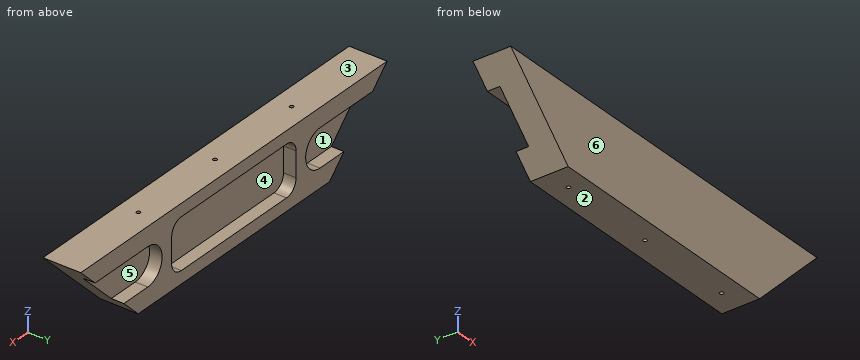
```python
from build123d import *

# Parameters (mm, degrees)
BOSS_EXTRUDE1_DEPTH = 15
CUT_EXTRUDE1_DEPTH  = 5
SKETCH3_R           = 0.75
CUT_EXTRUDE2_DEPTH  = 30
CUT_EXTRUDE3_DEPTH  = 5


with BuildPart() as part:
    # Sketch1 → Boss-Extrude1 (new body)
    with BuildSketch(Plane(origin=(0, 0, 0), x_dir=(1, 0, 0), z_dir=(0, 1, 0))):
        Polygon((0, 0), (160, 0), (130, 30), (30, 30), align=None)
    extrude(amount=BOSS_EXTRUDE1_DEPTH)

    # Sketch2 → Cut-Extrude1 (cut)
    with BuildSketch(Plane(origin=(0, 15, 0), x_dir=(1, 0, 0), z_dir=(0, 1, 0))):
        with BuildLine():
            Line((-5, 22.5), (35, 22.5))
            ThreePointArc((35, 22.5), (42.5, 15), (35, 7.5))
            Line((35, 7.5), (-5, 7.5))
            ThreePointArc((-5, 7.5), (-12.5, 15), (-5, 22.5))
        make_face()
        with BuildLine():
            Line((165, 22.5), (125, 22.5))
            ThreePointArc((125, 22.5), (117.5, 15), (125, 7.5))
            Line((125, 7.5), (165, 7.5))
            ThreePointArc((165, 7.5), (172.5, 15), (165, 22.5))
        make_face()
    extrude(amount=-CUT_EXTRUDE1_DEPTH, mode=Mode.SUBTRACT)

    # Sketch3 → Cut-Extrude2 (cut)
    with BuildSketch(Plane.XY):
        with Locations((80, 7.5)):
            Circle(SKETCH3_R)
        with Locations((40, 7.5)):
            Circle(SKETCH3_R)
        with Locations((120, 7.5)):
            Circle(SKETCH3_R)
    extrude(amount=-CUT_EXTRUDE2_DEPTH, mode=Mode.SUBTRACT)

    # Sketch4 → Cut-Extrude3 (cut)
    with BuildSketch(Plane(origin=(0, 15, 0), x_dir=(1, 0, 0), z_dir=(0, 1, 0))):
        with BuildLine():
            Line((52.5, 25), (107.5, 25))
            ThreePointArc((107.5, 25), (111.035533906, 23.535533906), (112.5, 20))
            Line((112.5, 20), (112.5, 10))
            ThreePointArc((112.5, 10), (111.035533906, 6.464466094), (107.5, 5))
            Line((107.5, 5), (52.5, 5))
            ThreePointArc((52.5, 5), (48.964466094, 6.464466094), (47.5, 10))
            Line((47.5, 10), (47.5, 20))
            ThreePointArc((47.5, 20), (48.964466094, 23.535533906), (52.5, 25))
        make_face()
    extrude(amount=-CUT_EXTRUDE3_DEPTH, mode=Mode.SUBTRACT)


solid = part.part
```
CAD build for the part. Positions are in the model's coordinates, mm. Face numbers are marked on the shaded views. A direction names the side the tool comes from. Coordinates: 2 decimals unless noted, no trailing zeros. Order: outer loops, then holes, each group sorted by start corner. A loop starts at its lowest first (then second) coordinate and runs counter-clockwise, first axis right, second up. Notation, with made-up numbers: M 8.25,-7 L 20.25,-7 A14 cw 20.25,7 Z; hole C 76.5,62.25 d6. An arc over 180 degrees is marked long. Write each question's results on one line, items separated by ' | '. Start each with the question number.
Q1. Drill centre lines: probe 1 along Y at (x, z) = (80, -12.25); probe 2 along Y at (x, z) = (40, -22); probe 3 along Z at (x, y) = (95, 10.25). Where is each one in solid material? Low to high. Write a range as from..to.
Q2. Cut at D-D (z = -15). List the corners of the cut face in (x, y).
Q3. Cut at C-C (z = -26.5). List the corners of the cut face in (x, y).
Q4. Pull direction Z, two halves, no side cores. Call the marked faces 1, 2 and 3: +Z half, -Z half, draft (parallel to the pull), parting line (faces both ways), or undercut.
Q5. Which spindle directions (+Z, -Z, +X, -X, +Y, -Y) get a long thin tool onto all of the face, cutting with end or side? Do the marked faces 4, 5 and 6. Say none if no direction does.
Q6. Cut at B-B (x = 93). List the corners of the cut face in (y, z).
Q7. Flat gauge pins, fed straight in: P1, Ø2, axis at y = 10.5, z = -10, coming from the -X side; P2, Ø5, axis at y = 11, z = -5.5, coming from the -X side; P3, Ø1.5, axis at x = 136, y = 12, coming from the -Z side; P4, Ø5.5, axis at x = 31, y = 13, coming from the +Z side. Where does each tip first touch, or does it go through?
Q8. Cut at A-A (z = -2.5). List the corners of the cut face in (x, y), then the cut area to 3 significant figures.
Found:
1) probe 1: 0..6.75, 8.25..10 | probe 2: 0..6.75, 8.25..15 | probe 3: -30..-25, -5..0
2) outline: M 15,0 L 145,0 L 145,10 L 117.5,10 L 117.5,15 L 112.5,15 L 112.5,10 L 47.5,10 L 47.5,15 L 42.5,15 L 42.5,10 L 15,10 Z; hole C 40,7.5 d1.5; hole C 80,7.5 d1.5; hole C 120,7.5 d1.5
3) outline: M 26.5,0 L 133.5,0 L 133.5,15 L 26.5,15 Z; hole C 40,7.5 d1.5; hole C 80,7.5 d1.5; hole C 120,7.5 d1.5
4) face 1: undercut | face 2: -Z half | face 3: +Z half
5) face 4: +Y | face 5: +X, +Y | face 6: +Z, -Z, +X, -X, -Y
6) outline: M 0,-30 L 15,-30 L 15,-25 L 10,-25 L 10,-5 L 15,-5 L 15,0 L 0,0 Z
7) P1: x = 9.13 | P2: x = 3 | P3: z = -24.75 | P4: z = 0
8) outline: M 2.5,0 L 157.5,0 L 157.5,15 L 2.5,15 Z; hole C 40,7.5 d1.5; hole C 80,7.5 d1.5; hole C 120,7.5 d1.5 | area: 2,320 mm²
